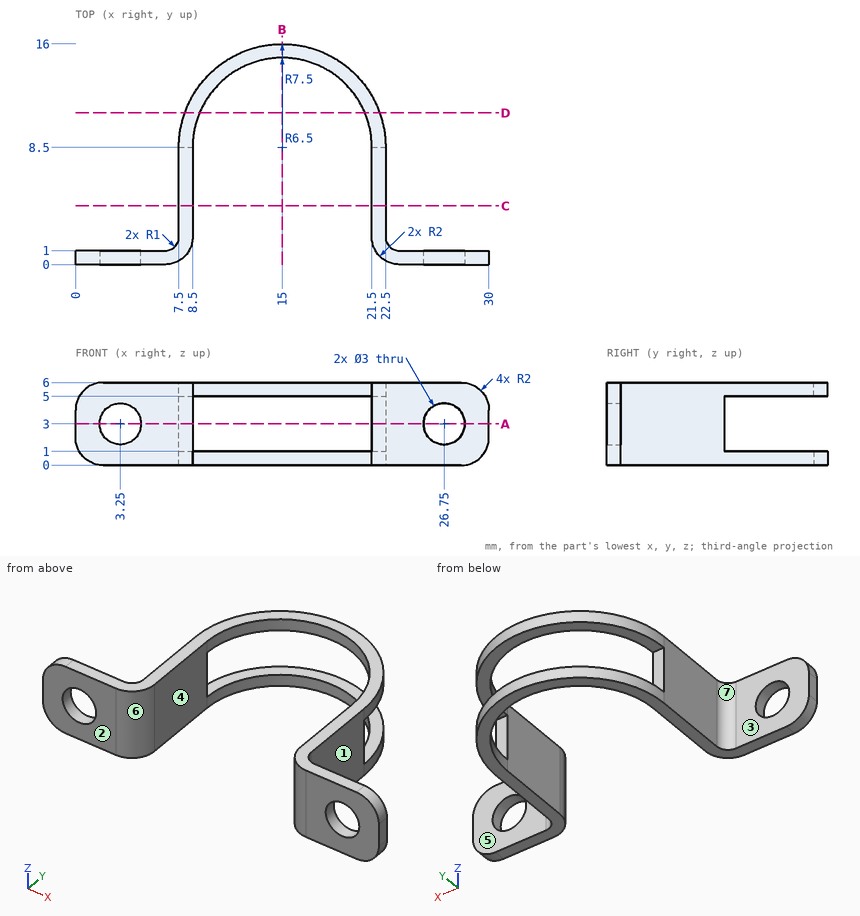
Answer from the drawing. Dimensions are ordinates in mm from the lowest x, y and z of the part. A direction names the side the tool comes from. Round coordinates to 2 decimals unless told otherwise and drop trailing zeros. Order: outer loops, then holes, each group sorted by start corner. A loop starts at its lowest first (then second) coordinate and runs counter-clockwise, first axis right, second up. Notation, with made-up numbers: (21.25, 67) -> (36.25, 67) arc R26 ccw to (36.25, 82) -> close; hole circle Ø11 at (-19, 66). An arc over 180 degrees is marked (long way). Answer as CSV lines item,"result".
Q1. A cutting plane is placed at A-A on z = 3. Determine the outline of the cut face in (x, y), plus the area to 3 significant figures.
Computed values:
outline,"(0, 0) -> (1.75, 0) -> (1.75, 1) -> (0, 1) -> close; (4.75, 0) -> (6.5, 0) arc R2 ccw to (8.5, 2) -> (8.5, 8.5) -> (7.5, 8.5) -> (7.5, 2) arc R1 cw to (6.5, 1) -> (4.75, 1) -> close; (21.5, 2) arc R2 ccw to (23.5, 0) -> (25.25, 0) -> (25.25, 1) -> (23.5, 1) arc R1 cw to (22.5, 2) -> (22.5, 8.5) -> (21.5, 8.5) -> close; (28.25, 0) -> (30, 0) -> (30, 1) -> (28.25, 1) -> close"
area,"24.7 mm^2"
Q2. A cutting plane is placed at B-B on x = 15. Determine the outline of the cut face in (y, z).
Computed values:
outline,"(15, 0) -> (16, 0) -> (16, 1) -> (15, 1) -> close; (15, 5) -> (16, 5) -> (16, 6) -> (15, 6) -> close"
Q3. Which of the six approach directions +Z, -Z, +X, -X, +Y, -Y give full straight-line access (tool end or side, diameter ignored) to the marked faces 1, 2, 3 and 4?
Computed values:
face 1,"+Z, -Z, +X, +Y"
face 2,"+Z, -Z, +X, -X, -Y"
face 3,"+Z, -Z, -X, +Y"
face 4,"+Z, -Z, -Y"
Q4. A cutting plane is placed at D-D on y = 11. Determine the outline of the cut face in (x, z).
Computed values:
outline,"(7.93, 0) -> (9, 0) -> (9, 1) -> (7.93, 1) -> close; (7.93, 5) -> (9, 5) -> (9, 6) -> (7.93, 6) -> close; (21, 0) -> (22.07, 0) -> (22.07, 1) -> (21, 1) -> close; (21, 5) -> (22.07, 5) -> (22.07, 6) -> (21, 6) -> close"
Q5. Given pin 1 (3 mm diameter, centred on y = 4.5, z = 3.5, fed in from -X); pin 2 (4 mm diameter, centred on x = 18.5, y = 10.5, fed in from -Z); pin 3 (1.8 mm diameter, centred on x = 2, z = 3.5, fed in from +Y); pin 4 (1.1 mm diameter, centred on x = 22, z = 3.5, fed in from +Y), each flat-ended and moving along its own axis, determine where each tip first touches the part or whether it passes through.
Computed values:
pin 1,"stops at x = 7.5"
pin 2,"passes through"
pin 3,"stops at y = 1"
pin 4,"stops at y = 8.5"
Q6. For a pull along X with two mould halves and no side action, classify the marked faces 5, 6 and 7 as +X half, -X half, draft (parallel to the pull), parting line (faces both ways), or undercut.
Computed values:
face 5,"draft"
face 6,"undercut"
face 7,"-X half"
Q7. Consider line 1 (Z direction, x = 3.25, y = 0.7); line 2 (X direction, y = 4.75, z = 0.9); line 3 (Y direction, x = 5.5, z = 0.7). Determine where each line is inside the solid, lowest interval first. Write a range as from..to.
Computed values:
line 1,"z = 0..1.5, 4.5..6"
line 2,"x = 7.5..8.5, 21.5..22.5"
line 3,"y = 0..1"
Q8. A cutting plane is placed at C-C on y = 4.25. Determine the outline of the cut face in (x, z).
Computed values:
outline,"(7.5, 0) -> (8.5, 0) -> (8.5, 6) -> (7.5, 6) -> close; (21.5, 0) -> (22.5, 0) -> (22.5, 6) -> (21.5, 6) -> close"
